Verification items for the finished model (mm, model axes). Give positions to 0.01 mm unless a question says otherwise; leave off trailing zeros. Write each loop counter-clockwise with the first axis right and the second up, starting at its lowest first coordinate (ties: lowest second). Pieces come first, ordered by that corner, then holes. Notation, with made-up numbers: (28.5, 59) - (35.5, 59) arc R11 ccw to (35.5, 63) - close; hole circle Ø7 at (1.5, 57). An arc over 180 degrees is marked (long way). Answer as a JSON object with one key per item and string values. Group by question number.
Item 1: Draft check along X on faces 1 (the face through (1.617, -1.479, -0.67)), 2 (the face through (-0.596, -0.493, -2.685)), 3 (the face through (1, -1, -3)). Enter one of: +X half, -X half, draft (parallel to the pull), parting line (faces both ways), or undercut.
Item 2: Sectioned sample at A-A, the plane z = 0. Record the boundary of the cut face in (x, y).
Item 3: Go/stop test with a flat-tipped pin: pin 1 (2.5 mm diameter, centred on x = 1.5, z = 1.5, fed in from +Y). Record where the tip stops, or that it passes through.
Item 4: Sectioned sample at D-D, the plane y = -2.75. Record the boundary of the cut face in (x, z).
Item 5: Sectioned sample at C-C, the plane y = -1.95. Record the boundary of the cut face in (x, z), and give its area (3 significant figures).
Item 6: Sectioned sample at B-B, the plane x = 0. Record the boundary of the cut face in (y, z).
Item 7: Scan lines: line 1 along Z through (x, y) = (0, -2.3); line 2 along Y through (x, z) = (2.5, -1.75); line 3 along X through (y, z) = (-0.8, 1.5). Record each from-to range of solid material in increasing order. Write a range as [from, to].
```python
from build123d import *

# Parameters (mm, degrees)
F0_R     = 2.75
F0_R_2   = 1.75
F1_DEPTH = 1
F2_R     = 4.5
F2_R_2   = 2.75
F2_R_3   = 1.75
F3_DEPTH = 2
F4_SIZE  = 0.4


with BuildPart() as f1:
    # F0 (on Front) → F1 (new body)
    with BuildSketch(Plane.XZ):
        Circle(F0_R)
        Circle(F0_R_2, mode=Mode.SUBTRACT)
    extrude(amount=F1_DEPTH)

    # F2 (on face) → F3 (join)
    with BuildSketch(Plane.XZ.offset(1)):
        Circle(F2_R)
        Circle(F2_R_2, mode=Mode.SUBTRACT)
        Circle(F2_R_2)
        Circle(F2_R_3, mode=Mode.SUBTRACT)
    extrude(amount=F3_DEPTH)

    # F4
    f4_edges = [f1.edges().sort_by_distance(p)[0] for p in [
        (-4.5, -3, 0),
        (-4.5, -1, 0),
    ]]
    chamfer(f4_edges, length=F4_SIZE)


solid = f1.part
```
Geometry check:
{
 "1": {"face 1": "undercut", "face 2": "parting line", "face 3": "draft"},
 "2": {"outline": "(-4.5, -2.6) - (-4.1, -3) - (-1.75, -3) - (-1.75, 0) - (-2.75, 0) - (-2.75, -1) - (-4.1, -1) - (-4.5, -1.4) - close; (1.75, -3) - (4.1, -3) - (4.5, -2.6) - (4.5, -1.4) - (4.1, -1) - (2.75, -1) - (2.75, 0) - (1.75, 0) - close"},
 "3": {"pin 1": "y = 0"},
 "4": {"outline": "circle Ø8.7 at (0, 0); hole circle Ø3.5 at (0, 0)"},
 "5": {"outline": "circle Ø9 at (0, 0); hole circle Ø3.5 at (0, 0)", "area": "54.0 mm^2"},
 "6": {"outline": "(-3, -4.1) - (-2.6, -4.5) - (-1.4, -4.5) - (-1, -4.1) - (-1, -2.75) - (0, -2.75) - (0, -1.75) - (-3, -1.75) - close; (-3, 1.75) - (0, 1.75) - (0, 2.75) - (-1, 2.75) - (-1, 4.1) - (-1.4, 4.5) - (-2.6, 4.5) - (-3, 4.1) - close"},
 "7": {"line 1": "[-4.5, -1.75], [1.75, 4.5]", "line 2": "[-3, -1]", "line 3": "[-2.3, -0.9], [0.9, 2.3]"}
}
